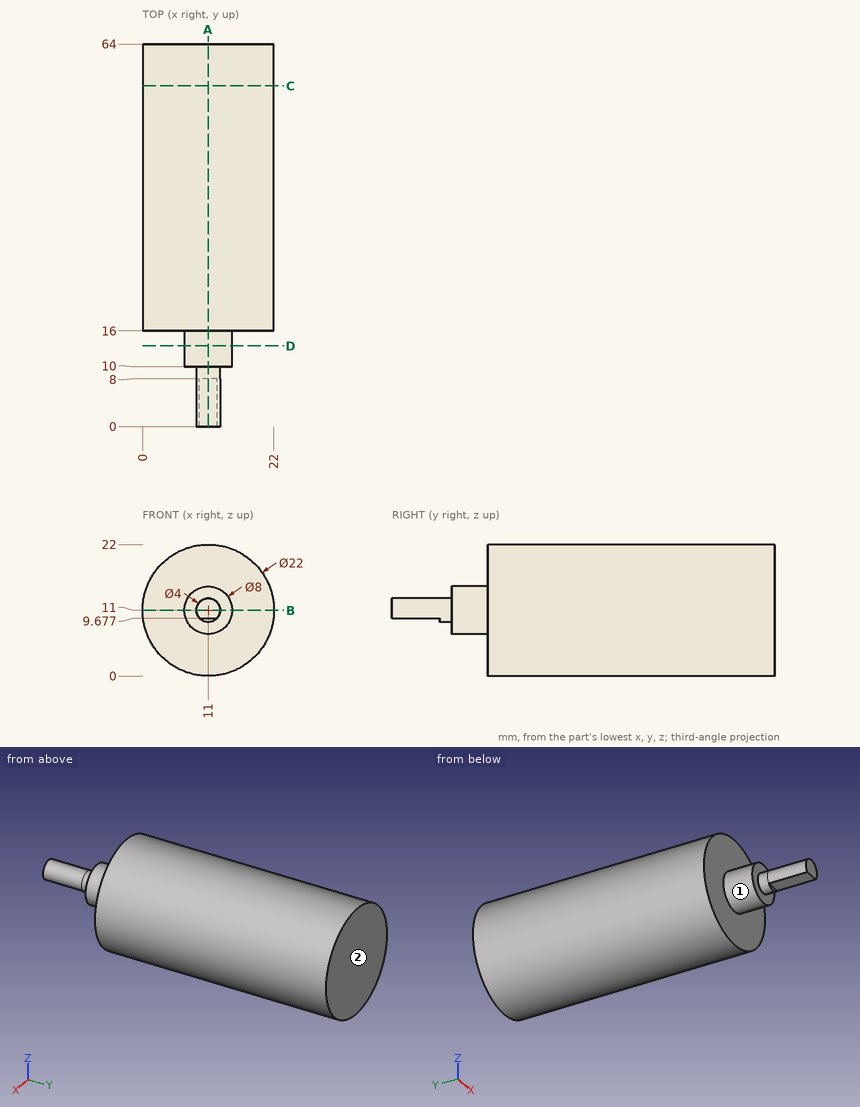
Design review of the part shown in the three views and the two pictorial views. Dimensions are in mm from the part's minimum x, y and z. A direction names the side the tool comes from. Coordinates: 2 decimals unless noted, no trailing zeros. Loops run counter-clockwise (first coordinate to the right, second up) from the corner with the lowest first, then second, coordinate; pieces in that order, holes last. Notation, with made-up numbers: (70, 75.25) - (82, 75.25) arc R14 ccw to (82, 94.25) - close; hole circle Ø3 at (8.25, -29.5). An arc over 180 degrees is marked (long way). Use a Markdown table: item, result. Add a question column.
Item 1: We need section A-A (x = 11). Give the boundary of the cut face in (y, z), and give its area (3 significant figures).
Item 2: Tool access review of the marked faces 1 and 2: name each direction out of +Z, -Z, +X, -X, +Y, -Y from which nothing blocks a thin tool from reaching the whole face with its end or side.
Item 3: We need section D-D (y = 13.5). Give the boundary of the cut face in (x, z).
Item 4: Insertion check: pin 1 Ø8 at (y, z) = (43.5, 10.5) entering from +X; pin 2 Ø5 at (y, z) = (55, 7) entering from +X; pin 3 Ø8 at (y, z) = (52, 17.5) entering from -X; pin 4 Ø10 at (y, z) = (48.5, 3.5) entering from +X. Each pin has a flat end and moves straight along its axis. Give the tip position at first contact, or say it passes through.
Item 5: For line 1 (Y direction, x = 7.25, z = 7.5); line 2 (Z direction, x = 11, y = 3); line 3 (X direction, y = 20, z = 15), list the stretches that pass through material, from the lowest coordinate up.
Item 6: We need section B-B (z = 11). Give the boundary of the cut face in (x, y).
Item 7: We need section C-C (y = 57). Give the boundary of the cut face in (x, z), and give its area (3 significant figures).
Results list:
| question | item | result |
|---|---|---|
| 1 | outline | (0, 9.68) - (8, 9.68) - (8, 9) - (10, 9) - (10, 7) - (16, 7) - (16, 0) - (64, 0) - (64, 22) - (16, 22) - (16, 15) - (10, 15) - (10, 13) - (0, 13) - close |
| 1 | area | 1,140 mm^2 |
| 2 | face 1 | -Y |
| 2 | face 2 | +Z, -Z, +X, -X, +Y |
| 3 | outline | circle Ø8 at (11, 11) |
| 4 | pin 1 | stops at x = 22 |
| 4 | pin 2 | stops at x = 21.9 |
| 4 | pin 3 | stops at x = 0.29 |
| 4 | pin 4 | stops at x = 21.71 |
| 5 | line 1 | y = 16 to 64 |
| 5 | line 2 | z = 9.68 to 13 |
| 5 | line 3 | x = 0.75 to 21.25 |
| 6 | outline | (0, 16) - (7, 16) - (7, 10) - (9, 10) - (9, 0) - (13, 0) - (13, 10) - (15, 10) - (15, 16) - (22, 16) - (22, 64) - (0, 64) - close |
| 7 | outline | circle Ø22 at (11, 11) |
| 7 | area | 380 mm^2 |
